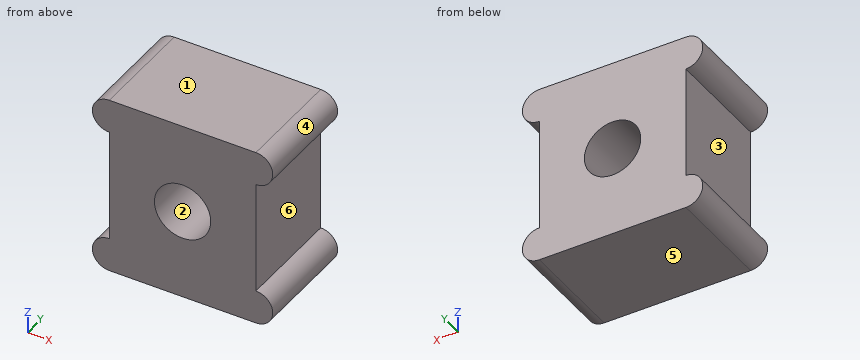
Autodesk Inventor part; units mm, degrees
ref_plane "YZ Plane" through (0, 0, 0) normal (1, 0, 0) x (0, 1, 0)
ref_plane "XZ Plane" through (0, 0, 0) normal (0, 1, 0) x (-1, 0, 0)
ref_plane "XY Plane" through (0, 0, 0) normal (0, 0, 1) x (1, 0, 0)
sketch "Sketch1" plane through (0, 0, 0) normal (0, 1, 0) x (-1, 0, 0)
  line L0 (6.5, 8) -> (-6.5, 8)
  line L1 (-6.5, 5) -> (-6.5, -5)
  line L2 (-6.5, -8) -> (6.5, -8)
  line L3 (6.5, -5) -> (6.5, 5)
  line L4 (6.5, 8) -> (-6.5, -8) construction
  line L5 (-6.5, 8) -> (6.5, -8) construction
  arc A0 (6.5, 5) -> (6.5, 8) centre (6.5, 6.5) ccw
  arc A1 (6.5, -8) -> (6.5, -5) centre (6.5, -6.5) ccw
  arc A2 (-6.5, -5) -> (-6.5, -8) centre (-6.5, -6.5) ccw
  arc A3 (-6.5, 8) -> (-6.5, 5) centre (-6.5, 6.5) ccw
  point P0 (0, 0)
  dimension "d1" = 16
extrude "Extrusion1" add sketch "Sketch1" along normal mid plane 9.5
sketch "Sketch2" plane through (0, 4.75, 0) normal (0, 1, 0) x (1, 0, 0)
  circle A0 centre (0, 0) radius 2.5
  dimension "d6" = 5
extrude "Extrusion2" cut sketch "Sketch2" against normal through all
properties part number "Varia"
Design review of the part built by this model. Coordinates are the model's own, in mm. Face numbers are marked on the shaded views. A direction names the side the tool comes from. Give positions to 0.01 mm unless a question says otherwise; leave off trailing zeros. Order: outer loops, then holes, each group sorted by start corner. A loop starts at its lowest first (then second) coordinate and runs counter-clockwise, first axis right, second up. Notation, with made-up numbers: (1, 89.5) - (10, 89.5) arc R11 ccw to (10, 97.5) - close; hole circle Ø11 at (-25.75, 8.5). An arc over 180 degrees is marked (long way). Use a Markdown table: item, result. Add a question column.
(1) Add section A-A on x = 0. Give the boundary of the cut face in (y, z).
(2) Add section B-B on z = -1.25. Give the boundary of the cut face in (x, y), then the cut area to 3 significant figures.
(3) Wall thickness on probe 1 along X at (y, z) = (-2.5, 0); probe 2 along Z at (x, y) = (0, 2.5); probe 3 along X at (y, z) = (3, -2): over which ranges is each line inside the solid? List them lowest first. Write a range as [from, to].
(4) Mouldability with a two-part tool opening along X and no side actions: class the marked faces 1, 2, 3 and 4 as +X half, -X half, draft (parallel to the pull), parting line (faces both ways), or undercut.
(5) Add section D-D on z = -4. Give the boundary of the cut face in (x, y), then the cut area to 4 significant figures.
(6) Clearance check with a flat-ended pin moving along its axis: P1, Ø4, axis at y = 0, z = 2, coming from the +X side. State where the tip first meets the part, or that it passes through.
(7) Add section C-C on y = -2.5. Give the boundary of the cut face in (x, z), then the cut area to 3 significant figures.
(8) Machinability: for the marked faces 5 and 6, which of the approach directions +Z, -Z, +X, -X, +Y, -Y give a long, thin tool a straight path to every point of the face, cutting with its end or side? Answer none if there is none.
Report:
| question | item | result |
|---|---|---|
| 1 | outline | (-4.75, -8) - (4.75, -8) - (4.75, -2.5) - (-4.75, -2.5) - close; (-4.75, 2.5) - (4.75, 2.5) - (4.75, 8) - (-4.75, 8) - close |
| 2 | outline | (-6.5, -4.75) - (-2.17, -4.75) - (-2.17, 4.75) - (-6.5, 4.75) - close; (2.17, -4.75) - (6.5, -4.75) - (6.5, 4.75) - (2.17, 4.75) - close |
| 2 | area | 82.4 mm² |
| 3 | probe 1 | x = [-6.5, -2.5], [2.5, 6.5] |
| 3 | probe 2 | z = [-8, -2.5], [2.5, 8] |
| 3 | probe 3 | x = [-6.5, -1.5], [1.5, 6.5] |
| 4 | face 1 | draft |
| 4 | face 2 | undercut |
| 4 | face 3 | -X half |
| 4 | face 4 | +X half |
| 5 | outline | (-6.5, -4.75) - (6.5, -4.75) - (6.5, 4.75) - (-6.5, 4.75) - close |
| 5 | area | 123.5 mm² |
| 6 | P1 | stops at x = 6.5 |
| 7 | outline | (-6.5, -8) - (6.5, -8) arc R1.5 ccw to (6.5, -5) - (6.5, 5) arc R1.5 ccw to (6.5, 8) - (-6.5, 8) arc R1.5 ccw to (-6.5, 5) - (-6.5, -5) arc R1.5 ccw to start; hole circle Ø5 at (0, 0) |
| 7 | area | 203 mm² |
| 8 | face 5 | -Z, +X, -X, +Y, -Y |
| 8 | face 6 | +X, +Y, -Y |
